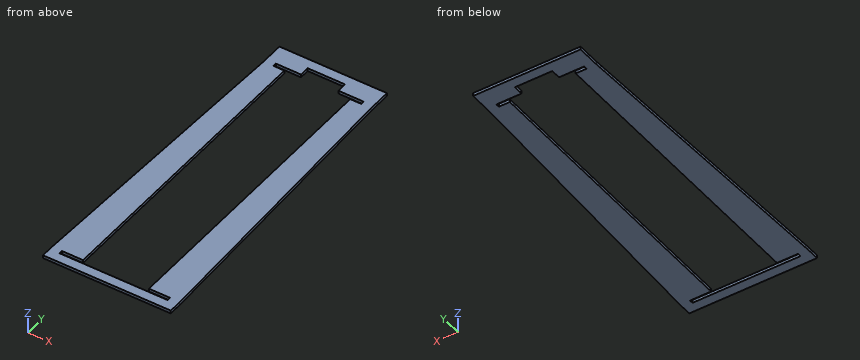
Autodesk Inventor part; units mm, degrees
ref_plane "YZ Plane" through (0, 0, 0) normal (1, 0, 0) x (0, 1, 0)
ref_plane "XZ Plane" through (0, 0, 0) normal (0, 1, 0) x (-1, 0, 0)
ref_plane "XY Plane" through (0, 0, 0) normal (0, 0, 1) x (1, 0, 0)
ref_plane "Work Plane1" through (-10, 297.2462, 0) normal (0, 0, 1) x (0, -1, 0)
ref_plane "Work Plane2" through (-53.2, 294.1262, 848.1435) normal (1, 0, 0) x (0, 0.6133, 0.7899)
sketch "Sketch1" plane through (-10, 297.2462, 0) normal (0, 0, 1) x (0, -1, 0)
  line L0 (94.5216, -24.7) -> (0, -24.7)
  line L1 (0, 0) -> (0, -24.7)
  line L2 (0, 0) -> (307.2462, 0)
  line L3 (307.2462, -10.6) -> (307.2462, 0)
  line L4 (307.2462, -10.6) -> (94.5216, -10.6)
  line L5 (94.5216, -10.6) -> (94.5216, -24.7)
  line L6 (89.5216, -75.8) -> (297.2462, -75.8)
  line L7 (297.2462, -75.8) -> (297.2462, -10.6)
  line L8 (307.2462, -10.6) -> (297.2462, -10.6)
  line L9 (307.2462, -10.6) -> (307.2462, -86.4)
  line L10 (0, -86.4) -> (307.2462, -86.4)
  line L11 (0, -86.4) -> (0, -61.7)
  line L12 (89.5216, -61.7) -> (0, -61.7)
  line L13 (89.5216, -75.8) -> (89.5216, -61.7)
  line L14 (297.2462, 10) -> (294.2462, 10)
  line L15 (297.2462, 10) -> (297.2462, 20)
  line L16 (297.2462, 20) -> (294.2462, 20)
  line L17 (294.2462, 10) -> (294.2462, 20)
  line L18 (297.2462, 10) -> (294.2462, 10)
  line L19 (0, 0) -> (0, 10)
  line L20 (0, 10) -> (-3, 10)
  line L21 (-3, 0) -> (-3, 10)
  line L22 (0, 0) -> (-3, 0)
  line L23 (0, -24.7) -> (-3, -24.7)
  line L24 (307.2462, 0) -> (307.2462, 20)
  line L25 (307.2462, 20) -> (297.2462, 20)
  line L26 (294.2462, 20) -> (0, 10)
  line L27 (-13, -24.7) -> (-3, -24.7)
  line L28 (-3, -24.7) -> (-3, 0)
  line L29 (-3, 10) -> (-13, 10)
  line L30 (-13, 10) -> (-13, -24.7)
  line L31 (297.2462, -43.2) -> (307.2462, -43.2)
  line L32 (297.2462, 10) -> (297.2462, -10.6)
  line L33 (294.2462, 10) -> (294.2462, -10.6)
  line L34 (94.5216, -10.6) -> (0, -10.6)
  line L35 (-89.0492, -43.2) -> (373.2954, -43.2) construction
  line L36 (-13, 10) -> (-23, 10)
  line L37 (-23, 10) -> (-23, -43.2)
  line L38 (-13, -24.7) -> (-13, -43.2)
  line L39 (-23, -43.2) -> (-13, -43.2)
  line L40 (297.4962, 10.25) -> (297.4962, -43.2)
  line L41 (297.4962, 10.25) -> (293.9962, 10.25)
  line L42 (293.9962, 10.25) -> (293.9962, -10.6)
  line L43 (0.25, 0.25) -> (0.25, -24.7)
  line L44 (-3.25, 0.25) -> (-3.25, -24.7)
  line L45 (-3.25, 0.25) -> (0.25, 0.25)
  point P0 (-3, 0.25)
  point P1 (0, 0.25)
  point P2 (0.25, -10.6)
  point P3 (297.4962, -43.2)
  dimension "d1" = 10
  dimension "d2" = 10
  dimension "d5" = 0.25
  dimension "d6" = 0.25
  dimension "d7" = 0.25
  dimension "d8" = 0.25
  dimension "d9" = 0.25
  dimension "d10" = 0.25
extrude "Extrusion1" add sketch "Sketch1" along normal blind 3 contours L34 L43 L2 L42 L4 | L43 L45 L19 L26 L17 L41 L42 L2 | L27 L30 L29 L21 L45 L44 | L45 L21 L20 L19 | L38 L39 L37 L36 L30 | L40 L2 L3 L4 | L4 L9 L31 L40 | L17 L16 L15 L41 | L40 L41 L15 L25 L24 L2
mirror "Mirror1" about plane through (-53.2, 294.1262, 848.1435) normal (1, 0, 0)
sketch "Sketch2" plane through (-10, 297.2462, 3) normal (0, 0, 1) x (1, 0, 0)
  line L0 (20, -307.2462) -> (-106.4, -307.2462)
  line L1 (20, -307.2462) -> (20, -294.2462)
  line L2 (20, -294.2462) -> (10, 0)
  line L3 (10, 0) -> (10, 23)
  line L4 (10, 23) -> (-96.4, 23)
  line L5 (-96.4, 0) -> (-96.4, 23)
  line L6 (-106.4, -294.2462) -> (-96.4, 0)
  line L7 (-106.4, -307.2462) -> (-106.4, -294.2462)
  line L8 (-75.8, -0.25) -> (-75.8, -293.9962)
  line L9 (-61.7, 13) -> (-61.7, 3.25)
  line L10 (-24.7, 13) -> (-61.7, 13)
  line L11 (-24.7, 13) -> (-24.7, 3.25)
  line L12 (-10.6, -0.25) -> (-10.6, -293.9962)
  line L13 (10.25, -297.4962) -> (-96.65, -297.4962)
  line L14 (-96.65, -293.9962) -> (-96.65, -297.4962)
  line L15 (-75.8, -293.9962) -> (-96.65, -293.9962)
  line L16 (-86.65, -0.25) -> (-75.8, -0.25)
  line L17 (-86.65, 3.25) -> (-86.65, -0.25)
  line L18 (-61.7, 3.25) -> (-86.65, 3.25)
  line L19 (-24.7, 3.25) -> (0.25, 3.25)
  line L20 (0.25, 3.25) -> (0.25, -0.25)
  line L21 (0.25, -0.25) -> (-10.6, -0.25)
  line L22 (-10.6, -293.9962) -> (10.25, -293.9962)
  line L23 (10.25, -293.9962) -> (10.25, -297.4962)
  point P0 (10, -297.2462)
equation "\"d6\" = d5"
equation "\"d7\" = d5"
equation "\"d8\" = d5"
equation "\"d9\" = d5"
equation "\"d10\" = d5"
properties part number "Upper Stand Bracket" material "Wood (Oak)"
Geometry: final body of the model. Coordinates: model frame, mm. Coordinates: 2 decimals unless noted, no trailing zeros. Order: outer loops, then holes, each group sorted by start corner. A loop starts at its lowest first (then second) coordinate and runs counter-clockwise, first axis right, second up. Notation, with made-up numbers: M 81,55 L 136,55 A16 ccw 136,85 Z; hole C 10.25,-15 d5. An arc over 180 degrees is marked long. Answer as CSV lines item,"result".
Q1. Section C-C on y = 246. Return the cut outline in (x, z), and give its area (3 significant figures).
Answers:
outline,"M -108.14,0 L -85.8,0 L -85.8,3 L -108.14,3 Z; M -20.6,0 L 1.74,0 L 1.74,3 L -20.6,3 Z"
area,"134 mm^2"
Q2. Line query: probe 1 along Y at (x, z) = (-94, 1.9); probe 2 along Y at (x, z) = (-36.5, 1.4); probe 3 along Y at (x, z) = (-85.5, 1.85). Output: solid intervals per line, ascending. Write a range as [from, to].
Answers:
probe 1,"y = [-10, -0.25], [3.25, 297], [300.5, 320.25]"
probe 2,"y = [-10, -0.25], [310.25, 320.25]"
probe 3,"y = [-10, -0.25], [300.5, 320.25]"
Q3. Section A-A on y = 101. Return the cut outline in (x, z).
Answers:
outline,"M -113.07,0 L -85.8,0 L -85.8,3 L -113.07,3 Z; M -20.6,0 L 6.67,0 L 6.67,3 L -20.6,3 Z"
Q4. First-contact query: P1, Ø1, axis at y = 212, z = 0.5, coming from the +X side; P2, Ø1.5, axis at y = 298, z = 2, coming from the +X side; P3, Ø0.9, axis at y = 157, z = 1.5, coming from the -X side. Flat tips, straight axial feed; report the tip coordinate or a pass-through.
Answers:
P1,"stops at x = 2.91"
P2,"stops at x = 0"
P3,"stops at x = -111.18"
Q5. Section B-B on z = 2.05. Return the cut outline in (x, y).
Answers:
outline,"M -116.4,-10 L 10,-10 L 10,3 L 0,297.25 L 0,320.25 L -106.4,320.25 L -106.4,297.25 L -116.4,3 Z; hole M -106.65,-0.25 L 0.25,-0.25 L 0.25,3.25 L -20.6,3.25 L -20.6,297 L -9.75,297 L -9.75,300.5 L -34.7,300.5 L -34.7,310.25 L -71.7,310.25 L -71.7,300.5 L -96.65,300.5 L -96.65,297 L -85.8,297 L -85.8,3.25 L -106.65,3.25 Z"
